The model under review builds one solid part; all positions refer to its coordinate system, in mm. A direction names the side the tool comes from. Give positions to 0.01 mm unless a question says otherwise; leave off trailing zeros. Loops run counter-clockwise (first coordinate to the right, second up) from the corner with the lowest first, then second, coordinate; pieces in that order, holes last. Notation, with made-up numbers: M 49.5,-35.5 L 86.5,-35.5 A24 cw 86.5,-1.5 Z; hole C 74,61.5 d2. An arc over 180 degrees is marked long. Return JSON: item names as keys, results as strings.
```python
from build123d import *

# Parameters (mm, degrees)
SKETCH_1_W          = 200
SKETCH_1_H          = 100
EXTRUDE_1_DEPTH     = 30
SKETCH_2_R          = 4.5
SKETCH_2_R_2        = 8
CUT_EXTRUDE_1_DEPTH = 226.610283454
SKETCH_3_R          = 4.5
CUT_EXTRUDE_2_DEPTH = 226.610283454
SKETCH_4_R          = 6.5
CUT_EXTRUDE_3_DEPTH = 50
SKETCH_5_R          = 6.5
CUT_EXTRUDE_4_DEPTH = 15
SKETCH_6_R          = 12
CUT_EXTRUDE_5_DEPTH = 15


with BuildPart() as part:
    # 草图1 → 凸台-拉伸1 (new body)
    with BuildSketch(Plane.XY):
        with Locations((100, 50)):
            Rectangle(SKETCH_1_W, SKETCH_1_H)
    extrude(amount=EXTRUDE_1_DEPTH)

    # 草图2 → 切除-拉伸1 (cut, through all)
    with BuildSketch(Plane.XY.offset(30)):
        with Locations((20, 25)):
            Circle(SKETCH_2_R)
        with Locations((100, 25)):
            Circle(SKETCH_2_R_2)
        with Locations((180, 25)):
            Circle(SKETCH_2_R)
    extrude(amount=-CUT_EXTRUDE_1_DEPTH, mode=Mode.SUBTRACT)

    # 草图3 → 切除-拉伸2 (cut, through all)
    with BuildSketch(Plane.XZ):
        with Locations(Location((60, 15, 0), (0, 0, 270))):
            Circle(SKETCH_3_R)
        with Locations(Location((140, 15, 0), (0, 0, 270))):
            Circle(SKETCH_3_R)
    extrude(amount=-CUT_EXTRUDE_2_DEPTH, mode=Mode.SUBTRACT)

    # 草图4 → 切除-拉伸3 (cut)
    with BuildSketch(Plane.XZ):
        with Locations(Location((60, 15, 0), (0, 0, 270))):
            Circle(SKETCH_4_R)
        with Locations(Location((140, 15, 0), (0, 0, 270))):
            Circle(SKETCH_4_R)
    extrude(amount=-CUT_EXTRUDE_3_DEPTH, mode=Mode.SUBTRACT)

    # 草图5 → 切除-拉伸4 (cut)
    with BuildSketch(Plane.XY.offset(30)):
        with Locations((20, 25)):
            Circle(SKETCH_5_R)
        with Locations((180, 25)):
            Circle(SKETCH_5_R)
    extrude(amount=-CUT_EXTRUDE_4_DEPTH, mode=Mode.SUBTRACT)

    # 草图6 → 切除-拉伸5 (cut)
    with BuildSketch(Plane(origin=(0, 0, 0), x_dir=(-1, 0, 0), z_dir=(0, 0, -1))):
        with Locations((-100, 25)):
            Circle(SKETCH_6_R)
    extrude(amount=-CUT_EXTRUDE_5_DEPTH, mode=Mode.SUBTRACT)


solid = part.part
```
1) Consider section C-C on y = 80. Write out the cut boundary in (x, z).
From the geometry:
{"outline": "M 0,0 L 200,0 L 200,30 L 0,30 Z; hole C 60,15 d9; hole C 140,15 d9"}
2) Consider section B-B on x = 60. Write out the cut boundary in (y, z), then the cut area to 3 significant figures.
From the geometry:
{"outline": "M 0,0 L 100,0 L 100,10.5 L 50,10.5 L 50,8.5 L 0,8.5 Z; M 0,21.5 L 50,21.5 L 50,19.5 L 100,19.5 L 100,30 L 0,30 Z", "area": "1,900 mm²"}
3) Insertion check: pin 1 (10.5 mm diameter, centred on x = 143, z = 12, fed in from -Y); pin 2 (11.5 mm diameter, centred on x = 180, y = 25, fed in from +Z); pin 3 (11.5 mm diameter, centred on x = 60, z = 15, fed in from -Y). Each pin has a flat end and moves straight along its axis. Give the tip position at first contact, or say it passes through.
From the geometry:
{"pin 1": "y = 0", "pin 2": "z = 15", "pin 3": "y = 50"}
4) Tool access review of faces 5 (the face through (18.46, 29.42, 15)), 6 (the face through (184.292, 26.352, 7.605)), 7 (the face through (92, 23, 15)), 8 (the face through (99, 51, 0)), 9 (the face through (61.54, 50, 19.42)): name each direction out of +Z, -Z, +X, -X, +Y, -Y from which nothing blocks a thin tool from reaching the whole face with its end or side.
From the geometry:
{"face 5": "+Z", "face 6": "+Z, -Z", "face 7": "-Z", "face 8": "-Z, +X, -X, +Y, -Y", "face 9": "-Y"}
5) Wall thickness on L1, parallel to Y at x = 100, z = 11; L2, parallel to X at y = 83, z = 15; L3, parallel to X at y = 59.5, z = 17.75: over which ranges is each line inside the solid? List them lowest first. Write a range as from..to.
From the geometry:
{"L1": "0..13, 37..100", "L2": "0..55.5, 64.5..135.5, 144.5..200", "L3": "0..56.44, 63.56..136.44, 143.56..200"}
6) The part is to be moulded in two halves that separate along X. For faces 1 (the face through (109.523, 17.698, 7.395)), 2 (the face through (200, 49, 15)), 3 (the face through (144.42, 50, 16.54)), 4 (the face through (99, 51, 30)), say which applies: released by +X, released by -X, zero draft, split by the parting line, or undercut.
From the geometry:
{"face 1": "undercut", "face 2": "released by +X", "face 3": "undercut", "face 4": "zero draft"}
7) Consider section A-A on z = 5.5. Write out the cut boundary in (x, y).
From the geometry:
{"outline": "M 0,0 L 200,0 L 200,100 L 0,100 Z; hole C 20,25 d9; hole C 100,25 d24; hole C 180,25 d9"}
8) Consider section D-D on z = 23.75. Write out the cut boundary in (x, y).
From the geometry:
{"outline": "M 0,0 L 200,0 L 200,100 L 0,100 Z; hole C 20,25 d13; hole C 100,25 d16; hole C 180,25 d13"}
